Autodesk Inventor part; units mm, degrees
ref_plane "YZ Plane" through (0, 0, 0) normal (1, 0, 0) x (0, 1, 0)
ref_plane "XZ Plane" through (0, 0, 0) normal (0, 1, 0) x (-1, 0, 0)
ref_plane "XY Plane" through (0, 0, 0) normal (0, 0, 1) x (1, 0, 0)
sketch "Sketch1" plane through (0, 0, 0) normal (0, 0, 1) x (1, 0, 0)
  arc A0 (0, 90) -> (77.9423, -45) centre (0, 0) ccw
  line L0 (0, 5) -> (0, 90)
  line L1 (77.9423, -45) -> (4.3301, -2.5)
  line L2 (0, 5) -> (0, 0)
  line L3 (0, 0) -> (4.3301, -2.5)
  line L4 (0, -167.6192) -> (0, 145.1192)
  dimension "d0" = 120
  dimension "d2" = 90
extrude "Extrusion1" add sketch "Sketch1" along normal blind 4
sketch "Sketch2" plane through (0, 0, 0) normal (0, 0, -1) x (-1, 0, 0)
  circle A0 centre (20.7055, 77.2741) radius 1.5
  circle A1 centre (6.9459, 39.3923) radius 1.5
  line L0 (0, 0) -> (0, 90)
  line L1 (20.7055, 77.2741) -> (0, 0)
  circle A2 centre (6.9725, 79.6956) radius 1.5
  line L2 (6.9725, 79.6956) -> (0, 0)
  line L3 (6.9459, 39.3923) -> (0, 0)
  dimension "d5" = 3
  dimension "d6" = 3
  dimension "d7" = 80
  dimension "d9" = 15
  dimension "d16" = 80
  dimension "d17" = 3
  dimension "d18" = 5
  dimension "d27" = 5
  dimension "d28" = 40
extrude "Extrusion2" cut sketch "Sketch2" against normal blind 10
pattern_circular "Circular Pattern1" count 12 over 220 about axis through (0, 0, 0) along (0, 0, 1) of "Extrusion2"
sketch "Sketch4" plane through (0, 0, 0) normal (0, 0, -1) x (-1, 0, 0)
  circle A0 centre (0, 0) radius 15
  dimension "d29" = 30
extrude "Extrusion4" cut sketch "Sketch4" against normal blind 10
sketch "Sketch5" plane through (0, 0, 4) normal (0, 0, 1) x (1, 0, 0)
  arc A0 (0, 15) -> (12.9904, -7.5) centre (0, 0) ccw
  line L0 (0, 0) -> (-30.7818, 84.5723)
  arc A1 (0, 90) -> (77.9423, -45) centre (0, 0) ccw
  line L1 (0, 0) -> (77.9423, -45)
  arc A2 (-30.7818, 84.5723) -> (77.9423, -45) centre (0, 0) ccw
  line L2 (0, 15) -> (0, 90)
  point P0 (12.9904, -7.5)
  point P1 (-5.1303, 14.0954)
  dimension "d32" = 20
extrude "Extrusion5" cut sketch "Sketch5" against normal blind 10 contours A0 L1 A1 L0
properties part number "cover2"
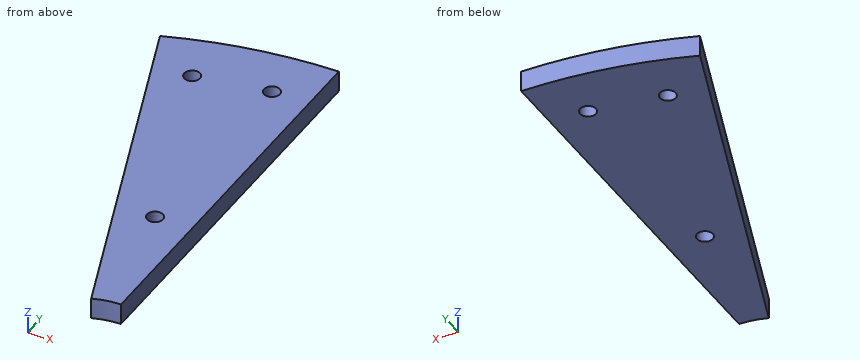
The model under review builds one solid part; all positions refer to its coordinate system, in mm. Coordinates: 2 decimals unless noted, no trailing zeros. Loops run counter-clockwise (first coordinate to the right, second up) from the corner with the lowest first, then second, coordinate; pieces in that order, holes last. Notation, with made-up numbers: (-28, 81.25) -> (-5, 81.25) arc R12 cw to (-5, 101.25) -> close; hole circle Ø6 at (-10, -1). An arc over 180 degrees is marked (long way). Answer as CSV lines item,"result".
Item 1: Insertion check: pin 1 (4 mm diameter, centred on x = -6.97, y = 79.7, fed in from -Z); pin 2 (1 mm diameter, centred on x = -14.5, z = 1.5, fed in from +Y); pin 3 (1.8 mm diameter, centred on x = -6.95, y = 39.39, fed in from -Z). Each pin has a flat end and moves straight along its axis. Give the tip position at first contact, or say it passes through.
Results below:
pin 1,"stops at z = 0"
pin 2,"stops at y = 88.9"
pin 3,"passes through"
Item 2: For L1, parallel to X at y = 78.5, z = 1.9; L2, parallel to X at y = 77.5, z = 1.35; L3, parallel to X at y = 46.5, z = 3.3, list the stretches that pass through material, from the lowest coordinate up.
Results below:
L1,"x = -28.57 to -21.57, -19.84 to -7.88, -6.07 to 0"
L2,"x = -28.21 to -22.19, -19.22 to 0"
L3,"x = -16.92 to 0"
Item 3: Take a section at A-A, the plane x = -21. State the section outline as (y, z) points.
Results below:
outline,"(57.7, 0) -> (75.8, 0) -> (75.8, 4) -> (57.7, 4) -> close; (78.74, 0) -> (87.52, 0) -> (87.52, 4) -> (78.74, 4) -> close"
Item 4: Take a section at D-D, the plane x = -26. State the section outline as (y, z) points, and give its area (3 significant figures).
Results below:
outline,"(71.43, 0) -> (86.16, 0) -> (86.16, 4) -> (71.43, 4) -> close"
area,"58.9 mm2"
Item 5: Take a section at C-C, the plane y = 51.5. State the section outline as (x, z) points, and give its area (3 significant figures).
Results below:
outline,"(-18.74, 0) -> (0, 0) -> (0, 4) -> (-18.74, 4) -> close"
area,"75.0 mm2"
Item 6: Take a section at B-B, the plane z = 2.15. State the section outline as (x, y) points.
Results below:
outline,"(-30.78, 84.57) -> (-5.13, 14.1) arc R15 cw to (0, 15) -> (0, 90) arc R90 ccw to start; hole circle Ø3 at (-20.71, 77.27); hole circle Ø3 at (-6.97, 79.7); hole circle Ø3 at (-6.95, 39.39)"
